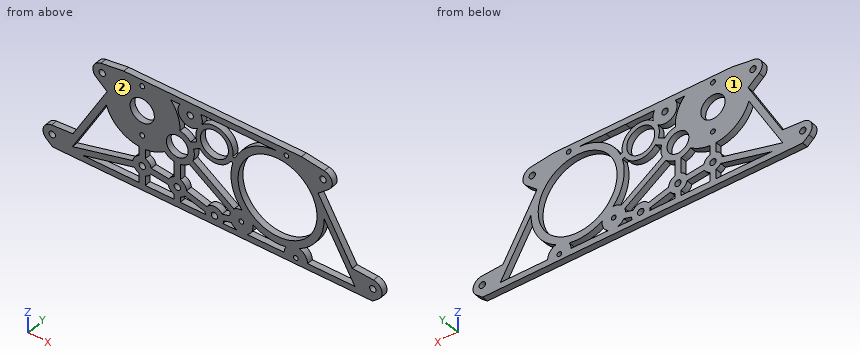
from build123d import *

# Parameters (mm, degrees)
SKETCH1_R           = 12.3825
SKETCH1_R_2         = 2.4892
SKETCH1_R_3         = 11.1252
SKETCH1_R_4         = 14.3002
SKETCH1_R_5         = 2.413
SKETCH1_R_6         = 40.3225
SKETCH1_R_7         = 3.2639
BOSS_EXTRUDE1_DEPTH = 6.35
SKETCH3_R           = 3.2639
SKETCH3_R_2         = 3.258583446
CUT_EXTRUDE2_DEPTH  = 233.226149567


with BuildPart() as part:
    # Sketch1 → Boss-Extrude1 (new body)
    with BuildSketch(Plane(origin=(0, 0, 0), x_dir=(1, 0, 0), z_dir=(0, 1, 0))):
        Polygon((-155.087712155, 84.29625), (-89.463193808, -29.36875), (150.668810904, -29.36875), (216.293329251, 84.29625), align=None)
        with Locations(Location((-41.275, 2.38125, 0), (0, 0, 270))):
            Circle(SKETCH1_R, mode=Mode.SUBTRACT)
        with Locations(Location((-41.275, 27.78125, 0), (0, 0, 270))):
            Circle(SKETCH1_R_2, mode=Mode.SUBTRACT)
        with Locations(Location((-41.275, -23.01875, 0), (0, 0, 270))):
            Circle(SKETCH1_R_2, mode=Mode.SUBTRACT)
        with Locations(Location((-5.496024757, 21.654924548, 0), (0, 0, 270))):
            Circle(SKETCH1_R_3, mode=Mode.SUBTRACT)
        with Locations(Location((32.48383617, 1.11125, 0), (0, 0, 270))):
            Circle(SKETCH1_R_4, mode=Mode.SUBTRACT)
        with Locations(Location((60.01758652, 67.406835627, 0), (0, 0, 270))):
            Circle(SKETCH1_R_5, mode=Mode.SUBTRACT)
        with Locations(Location((115.607306669, 77.94625, 0), (0, 0, 270))):
            Circle(SKETCH1_R_5, mode=Mode.SUBTRACT)
        with Locations(Location((105.955591438, -23.01875, 0), (0, 0, 270))):
            Circle(SKETCH1_R_5, mode=Mode.SUBTRACT)
        with Locations(Location((96.939901816, 24.534144815, 0), (0, 0, 270))):
            Circle(SKETCH1_R_6, mode=Mode.SUBTRACT)
        with Locations(Location((-133.090666899, 71.59625, 0), (0, 0, 270))):
            Circle(SKETCH1_R_7, mode=Mode.SUBTRACT)
        with Locations(Location((-82.130845389, -16.66875, 0), (0, 0, 270))):
            Circle(SKETCH1_R_7, mode=Mode.SUBTRACT)
        with Locations(Location((194.296283995, 71.59625, 0), (0, 0, 270))):
            Circle(SKETCH1_R_7, mode=Mode.SUBTRACT)
        with Locations(Location((143.336462485, -16.66875, 0), (0, 0, 270))):
            Circle(SKETCH1_R_7, mode=Mode.SUBTRACT)
    extrude(amount=BOSS_EXTRUDE1_DEPTH)

    # Sketch3 → Cut-Extrude2 (cut, through all)
    with BuildSketch(Plane(origin=(0, 6.35, 0), x_dir=(1, 0, 0), z_dir=(0, 1, 0))):
        with BuildLine():
            Line((216.293329251, 84.29625), (194.094002759, 84.29625))
            Line((194.094002759, 84.29625), (200.482952973, 78.838539138))
            ThreePointArc((200.482952973, 78.838539138), (203.338674486, 68.602790594), (194.939381575, 62.092984745))
            Line((194.939381575, 62.092984745), (173.299400368, 60.628580757))
            Line((173.299400368, 60.628580757), (138.359146632, 0.110286058))
            Line((138.359146632, 0.110286058), (149.523131463, -9.426460862))
            ThreePointArc((149.523131463, -9.426460862), (152.480247084, -19.336488408), (144.658083658, -26.101615019))
            Line((144.658083658, -26.101615019), (121.339417229, -29.36875))
            Line((121.339417229, -29.36875), (150.668810904, -29.36875))
            Line((150.668810904, -29.36875), (216.293329251, 84.29625))
        make_face()
        with BuildLine():
            Line((-139.277335877, 78.838539138), (-132.888385663, 84.29625))
            Line((-132.888385663, 84.29625), (-155.087712155, 84.29625))
            Line((-155.087712155, 84.29625), (-89.463193808, -29.36875))
            Line((-89.463193808, -29.36875), (-60.133800133, -29.36875))
            Line((-60.133800133, -29.36875), (-83.452466562, -26.101615019))
            ThreePointArc((-83.452466562, -26.101615019), (-91.274629988, -19.336488408), (-88.317514367, -9.426460862))
            Line((-88.317514367, -9.426460862), (-77.153529536, 0.110286058))
            Line((-77.153529536, 0.110286058), (-112.093783272, 60.628580757))
            Line((-112.093783272, 60.628580757), (-133.733764479, 62.092984745))
            ThreePointArc((-133.733764479, 62.092984745), (-142.13305739, 68.602790594), (-139.277335877, 78.838539138))
        make_face()
        with BuildLine():
            Line((47.814092291, -23.01875), (68.181438384, -23.083024918))
            Line((68.181438384, -23.083024918), (96.076321123, -23.083024918))
            ThreePointArc((96.076321123, -23.083024918), (70.568830934, -15.123228341), (53.3627184, 5.320355219))
            Line((53.3627184, 5.320355219), (51.222267729, 4.542530038))
            ThreePointArc((51.222267729, 4.542530038), (41.625748882, -15.601856592), (19.486846811, -12.816447857))
            ThreePointArc((19.486846811, -12.816447857), (20.025058188, -18.04104949), (18.349161012, -23.01875))
            Line((18.349161012, -23.01875), (47.814092291, -23.01875))
        make_face()
        with BuildLine():
            ThreePointArc((65.624420624, 77.94625), (70.839432321, 72.447023863), (71.692940222, 64.916462174))
            ThreePointArc((71.692940222, 64.916462174), (88.068575871, 71.325599173), (105.653728832, 71.355185424))
            ThreePointArc((105.653728832, 71.355185424), (104.176172512, 74.504591113), (103.669306669, 77.94625))
            Line((103.669306669, 77.94625), (65.624420624, 77.94625))
        make_face()
        with BuildLine():
            Line((49.053481172, 10.510684265), (51.193931844, 11.288509446))
            ThreePointArc((51.193931844, 11.288509446), (50.390005045, 34.596338197), (60.748765196, 55.491248283))
            ThreePointArc((60.748765196, 55.491248283), (56.315080015, 56.057505709), (52.400421048, 58.214739339))
            Line((52.400421048, 58.214739339), (10.400093309, 28.883502325))
            ThreePointArc((10.400093309, 28.883502325), (11.938221759, 22.647877037), (11.11803249, 16.277935796))
            Line((11.11803249, 16.277935796), (17.472938166, 12.840505779))
            ThreePointArc((17.472938166, 12.840505779), (33.885421031, 20.109619927), (49.053481172, 10.510684265))
        make_face()
        with BuildLine():
            Line((-12.26642072, -23.01875), (-2.911488672, -23.01875))
            ThreePointArc((-2.911488672, -23.01875), (-0.572987431, -7.472448155), (15.13161349, -6.750230017))
            ThreePointArc((15.13161349, -6.750230017), (13.456237349, 0.187679153), (14.451809556, 7.255232113))
            Line((14.451809556, 7.255232113), (8.09690388, 10.69266213))
            ThreePointArc((8.09690388, 10.69266213), (3.247440056, 6.539014741), (-2.771017966, 4.40635231))
            ThreePointArc((-2.771017966, 4.40635231), (-4.839844683, -10.233706554), (-12.26642072, -23.01875))
        make_face()
        with BuildLine():
            Line((-50.759436627, 58.498761805), (-112.546125373, 74.112060259))
            Line((-112.546125373, 74.112060259), (-77.968891343, 14.222534134))
            ThreePointArc((-77.968891343, 14.222534134), (-65.234805689, 32.590278174), (-44.45, 40.807504655))
            Line((-44.45, 40.807504655), (-44.45, 50.396621207))
            ThreePointArc((-44.45, 50.396621207), (-48.790085129, 53.524602513), (-50.759436627, 58.498761805))
        make_face()
        with BuildLine():
            Line((-44.45, 77.94625), (-101.800382387, 77.94625))
            Line((-101.800382387, 77.94625), (-49.203714213, 64.655240325))
            ThreePointArc((-49.203714213, 64.655240325), (-47.127274815, 66.891962457), (-44.45, 68.357133449))
            Line((-44.45, 68.357133449), (-44.45, 77.94625))
        make_face()
        with BuildLine():
            Line((175.965412948, 77.94625), (127.545306669, 77.94625))
            ThreePointArc((127.545306669, 77.94625), (125.262868019, 70.925852645), (119.288315712, 66.58992945))
            ThreePointArc((119.288315712, 66.58992945), (138.013120037, 48.640811318), (144.554546133, 23.541032766))
            Line((144.554546133, 23.541032766), (175.965412948, 77.94625))
        make_face()
        with BuildLine():
            Line((-8.671024757, 77.94625), (-38.1, 77.94625))
            Line((-38.1, 77.94625), (-38.1, 68.357133449))
            ThreePointArc((-38.1, 68.357133449), (-34.952622948, 66.501003479), (-32.735648144, 63.596485707))
            Line((-32.735648144, 63.596485707), (-14.789932822, 65.744151131))
            ThreePointArc((-14.789932822, 65.744151131), (-12.620150909, 69.981127052), (-8.671024757, 72.639006121))
            Line((-8.671024757, 72.639006121), (-8.671024757, 77.94625))
        make_face()
        with BuildLine():
            Line((23.503580049, 77.94625), (-2.321024757, 77.94625))
            Line((-2.321024757, 77.94625), (-2.321024757, 72.639006121))
            ThreePointArc((-2.321024757, 72.639006121), (0.215735977, 71.281178374), (2.231289861, 69.227792449))
            Line((2.231289861, 69.227792449), (22.973340196, 75.296693933))
            ThreePointArc((22.973340196, 75.296693933), (23.144028083, 76.640370087), (23.503580049, 77.94625))
        make_face()
        with BuildLine():
            Line((6.76434919, 34.08963954), (48.764676929, 63.420876554))
            ThreePointArc((48.764676929, 63.420876554), (48.260129345, 65.338492141), (48.079953972, 67.313170504))
            Line((48.079953972, 67.313170504), (40.338763738, 69.383696019))
            ThreePointArc((40.338763738, 69.383696019), (32.5947676, 65.246895995), (24.756521552, 69.202207551))
            Line((24.756521552, 69.202207551), (4.014471217, 63.133306067))
            ThreePointArc((4.014471217, 63.133306067), (2.126403616, 57.946989266), (-2.321024757, 54.678493879))
            Line((-2.321024757, 54.678493879), (-2.321024757, 38.826362497))
            ThreePointArc((-2.321024757, 38.826362497), (2.576882297, 37.139338581), (6.76434919, 34.08963954))
        make_face()
        with BuildLine():
            Line((-14.035376613, 59.43914162), (-31.981091935, 57.291476197))
            ThreePointArc((-31.981091935, 57.291476197), (-34.150873849, 53.054500276), (-38.1, 50.396621207))
            Line((-38.1, 50.396621207), (-38.1, 40.807504655))
            ThreePointArc((-38.1, 40.807504655), (-27.736533159, 38.483432585), (-18.400321213, 33.420044149))
            ThreePointArc((-18.400321213, 33.420044149), (-13.977947484, 36.919127544), (-8.671024757, 38.826362497))
            Line((-8.671024757, 38.826362497), (-8.671024757, 54.678493879))
            ThreePointArc((-8.671024757, 54.678493879), (-11.818401809, 56.534623849), (-14.035376613, 59.43914162))
        make_face()
        with BuildLine():
            ThreePointArc((41.196515027, 78.620256643), (41.719201203, 77.102270743), (41.979514016, 75.518061392))
            Line((41.979514016, 75.518061392), (49.720704249, 73.447535877))
            ThreePointArc((49.720704249, 73.447535877), (52.370619317, 76.57415457), (55.921852993, 78.620256643))
            Line((55.921852993, 78.620256643), (41.196515027, 78.620256643))
        make_face()
        with Locations(Location((-5.496024757, 63.65875, 0), (0, 0, 270))):
            Circle(SKETCH3_R)
        with Locations(Location((-41.275, 59.376877328, 0), (0, 0, 270))):
            Circle(SKETCH3_R)
        with Locations(Location((7.71883617, -16.66875, 0), (0, 0, 270))):
            Circle(SKETCH3_R_2)
        with Locations(Location((32.48383617, 74.77125, 0), (0, 0, 270))):
            Circle(SKETCH3_R)
    extrude(amount=-CUT_EXTRUDE2_DEPTH, mode=Mode.SUBTRACT)


solid = part.part
Model file for the job. Use its own axes, mm. Face numbers are marked on the shaded views. Give positions to 0.01 mm unless a question says otherwise; leave off trailing zeros. Order: outer loops, then holes, each group sorted by start corner. A loop starts at its lowest first (then second) coordinate and runs counter-clockwise, first axis right, second up. Notation, with made-up numbers: M 20,12.25 L 53,12.25 A14 ccw 53,27.25 Z; hole C 8,44 d1. An arc over 180 degrees is marked long. Put each result on its own line as item: value. Start each with the question number.
(1) Band-saw the part on B-B on y = 5. Count the separate pieces of the cut face and the enclosed holes in it, then the cut area to 3 significant figures.
(2) Band-saw the part on A-A on z = -47. Give the cut face in (x, y), then the cut area to 3 significant figures.
(3) Pin check, flat tips, straight feed: pin 1 Ø10 at (x, z) = (33, -14.5) entering from -Y; pin 2 Ø3 at (y, z) = (3.5, -73.5) entering from -X; pin 3 Ø2 at (y, z) = (5.5, -28) entering from +X; pin 4 Ø3 at (y, z) = (2, -45) entering from +X. Stop position of each tip, or through.
(4) Pull direction Y, two halves, no side cores. Call the marked faces 1 and 2: released by +Y, released by -Y, zero draft, split by the parting line, or undercut.
(5) Drill centre lines: L1, parallel to X at y = 0.75, z = -31; L2, parallel to Z at x = -55, y = 1; L3, parallel to Z at x = 54.5, y = 3.75. Where is each one in solid material? Low to high. Write a range as [from, to].
Results below:
1. separate pieces: 1
1. enclosed holes: 29
1. area: 15,100 mm2
2. outline: M -104.23,0 L -96.89,0 L -96.89,6.35 L -104.23,6.35 Z; M -44.45,0 L -38.1,0 L -38.1,6.35 L -44.45,6.35 Z; M -8.67,0 L -2.32,0 L -2.32,6.35 L -8.67,6.35 Z; M 25.25,0 L 36.34,0 L 36.34,6.35 L 25.25,6.35 Z; M 54.95,0 L 63.46,0 L 63.46,6.35 L 54.95,6.35 Z; M 130.42,0 L 138.93,0 L 138.93,6.35 L 130.42,6.35 Z; M 158.1,0 L 165.43,0 L 165.43,6.35 L 158.1,6.35 Z
2. area: 352 mm2
3. pin 1: stops at y = 0
3. pin 2: stops at x = -142.61
3. pin 3: stops at x = 155.04
3. pin 4: stops at x = 165.14
4. face 1: released by +Y
4. face 2: released by -Y
5. L1: x = [-94.99, -87.66], [-67.11, -11.53], [0.54, 13.43], [49.76, 57.14], [136.74, 144.12], [148.86, 156.19]
5. L2: z = [-84.3, -77.95], [-66.12, -59.57], [-38.41, 29.37]
5. L3: z = [-84.3, -78.62], [-77.99, -56.82], [-46.14, -2.92], [23.04, 29.37]
